Input: part model. Units: mm. Frame: model coordinates. Give positions to 0.01 mm unless a question says otherwise; leave off trailing zeros. Write each loop counter-clockwise with the first axis right and the second up, starting at its lowest first coordinate (ties: lowest second). Pieces come first, ordered by that corner, then holes. Notation, with made-up numbers: (-15, 10) - (1, 10) arc R9 cw to (1, 23) - close; hole circle Ø5 at (11, 67.25). An arc over 180 degrees is marked (long way). Answer as a JSON object with one key per item and string values. Group by question number.
from build123d import *

# Parameters (mm, degrees)
SKETCH1_W                  = 165.1
SKETCH1_H                  = 76.2
BOSS_EXTRUDE1_DEPTH        = 2.54
F_1_4_0_2500_DOWEL_HOLE1_D = 6.35


with BuildPart() as part:
    # Sketch1 → Boss-Extrude1 (new body)
    with BuildSketch(Plane.XY):
        Rectangle(SKETCH1_W, SKETCH1_H)
    extrude(amount=BOSS_EXTRUDE1_DEPTH)

    # 1/4 (0.2500) Dowel Hole1 (through all)
    with Locations(Plane(origin=(-50.512645238, 8.474787733, 2.54), x_dir=(1, 0, 0), z_dir=(0, 0, 1))):
        with Locations((0, 0), (41.154917852, -27.464087264), (82.739905764, 15.386269222)):
            Hole(F_1_4_0_2500_DOWEL_HOLE1_D / 2)


solid = part.part
1) Pin query (flat end, axial travel): P1, Ø5.5, axis at x = -50.51, y = 8.47, coming from the -Z side. Return the tip coordinate at first contact, or that it passes through.
2) Cut plane A-A on x = -51. Return the cut outline in (y, z), and give its area (3 significant figures).
3) Line query: line 1 along Y through (x, z) = (-9.5, 1.05); line 2 along Y through (x, z) = (30.5, 1.3); line 3 along X through (y, z) = (22, 0.25). Output: solid intervals per line, ascending. Write a range as from..to.
4) Mould query, pull axis Y, two halves, no side actions, for faces 1 (the face through (-1, 1, 2.54)), 2 (the face through (34.567, 26.007, 1.252)), 3 (the face through (-53.54, 9.43, 1.25)). Classes: +Y half, -Y half, draft (parallel to the pull), parting line (faces both ways), or undercut.
Filled in:
{
 "1": {"P1": "passes through"},
 "2": {"outline": "(-38.1, 0) - (5.34, 0) - (5.34, 2.54) - (-38.1, 2.54) - close; (11.61, 0) - (38.1, 0) - (38.1, 2.54) - (11.61, 2.54) - close", "area": "178 mm²"},
 "3": {"line 1": "y = -38.1..-22.16, -15.82..38.1", "line 2": "y = -38.1..21.2, 26.53..38.1", "line 3": "x = -82.55..29.65, 34.8..82.55"},
 "4": {"face 1": "draft", "face 2": "undercut", "face 3": "undercut"}
}
